Can you work these out from the model? Positions are in its coordinate system, mm. A direction names the side the tool comes from. Give positions to 0.01 mm unless a question says otherwise; leave off trailing zeros. Write each loop counter-clockwise with the first axis right and the second up, starting at its lowest first coordinate (ties: lowest second). Pieces come first, ordered by that corner, then holes.
from build123d import *

# Parameters (mm, degrees)
SKETCH1_R           = 76.2
SKETCH1_R_2         = 6.35
BOSS_EXTRUDE1_DEPTH = 2.413
SKETCH2_R           = 7.62
SKETCH2_R_2         = 6.35
BOSS_EXTRUDE3_DEPTH = 0.762
SKETCH4_R           = 76.257533764
CUT_EXTRUDE1_DEPTH  = 93.98
SKETCH5_R           = 1.016
CUT_EXTRUDE2_DEPTH  = 93.98


with BuildPart() as part:
    # Sketch1 → Boss-Extrude1 (new body)
    with BuildSketch(Plane.XY):
        Circle(SKETCH1_R)
        Circle(SKETCH1_R_2, mode=Mode.SUBTRACT)
    extrude(amount=BOSS_EXTRUDE1_DEPTH)

    # Sketch2 → Boss-Extrude3 (add)
    with BuildSketch(Plane.XY.offset(2.413)):
        with Locations(Location((0, 0, 0), (0, 0, 180))):
            Circle(SKETCH2_R)
        Circle(SKETCH2_R_2, mode=Mode.SUBTRACT)
    extrude(amount=BOSS_EXTRUDE3_DEPTH)

    # Sketch4 → Cut-Extrude1 (cut)
    with BuildSketch(Plane(origin=(0, 0, 0), x_dir=(-1, 0, 0), z_dir=(0, 0, -1))):
        Circle(SKETCH4_R)
        with BuildLine():
            Line((10.795, 13.97), (-10.795, 13.97))
            ThreePointArc((-10.795, 13.97), (-13.04006403, 14.89993597), (-13.97, 17.145))
            Line((-13.97, 17.145), (-13.97, 26.67))
            Line((-13.97, 26.67), (-18.20732863, 26.67))
            ThreePointArc((-18.20732863, 26.67), (-20.55370118, 20.591203739), (-23.658870968, 14.862752926))
            Line((-23.658870968, 14.862752926), (-4.737825132, -30.035944056))
            ThreePointArc((-4.737825132, -30.035944056), (0, -31.403636364), (4.737825132, -30.035944056))
            Line((4.737825132, -30.035944056), (23.658870968, 14.862752926))
            ThreePointArc((23.658870968, 14.862752926), (20.55370118, 20.591203739), (18.20732863, 26.67))
            Line((18.20732863, 26.67), (13.97, 26.67))
            Line((13.97, 26.67), (13.97, 17.145))
            ThreePointArc((13.97, 17.145), (13.04006403, 14.89993597), (10.795, 13.97))
        make_face(mode=Mode.SUBTRACT)
    extrude(amount=-CUT_EXTRUDE1_DEPTH, mode=Mode.SUBTRACT)

    # Sketch5 → Cut-Extrude2 (cut)
    with BuildSketch(Plane.XY.offset(2.413)):
        with Locations((-16.764, 23.241)):
            Circle(SKETCH5_R)
        with Locations((16.764, 23.241)):
            Circle(SKETCH5_R)
        with Locations((0, -28.575)):
            Circle(SKETCH5_R)
        with Locations((-5.5499, 8.7376)):
            Circle(SKETCH5_R)
        with Locations((5.5499, 8.7376)):
            Circle(SKETCH5_R)
    extrude(amount=-CUT_EXTRUDE2_DEPTH, mode=Mode.SUBTRACT)


solid = part.part
(1) Imagine slicing it at B-B, the plane y = 0. Write out the boundary of the cut face in (x, z) (3 decimals), plus the area to 3 significant figures.
Returned:
outline: (-17.395, 0) - (-6.35, 0) - (-6.35, 3.175) - (-7.62, 3.175) - (-7.62, 2.413) - (-17.395, 2.413) - close; (6.35, 0) - (17.395, 0) - (17.395, 2.413) - (7.62, 2.413) - (7.62, 3.175) - (6.35, 3.175) - close
area: 55.2 mm2
(2) Imagine slicing it at D-D, the plane x = -16.5. Write out the boundary of the cut face in (y, z), plus the area to 3 significant figures.
Returned:
outline: (-2.12, 0) - (22.26, 0) - (22.26, 2.41) - (-2.12, 2.41) - close; (24.22, 0) - (26.67, 0) - (26.67, 2.41) - (24.22, 2.41) - close
area: 64.7 mm2
(3) For faces 4 (the face through (-4.58, 9.04, 1.22)), 5 (the face through (0.992, -7.555, 2.789)), 6 (the face through (0, 13.97, 1)), which set-ups out of +Z, -Z, +X, -X, +Y, -Y let a thin tool reach every point of the face, with its end or its side?
Returned:
face 4: +Z, -Z
face 5: +Z
face 6: +Z, -Z, +Y
(4) Will these pins go through, and if not, where does the flat tip stop? P1, Ø1.9, axis at y = 21.5, z = 1, coming from the -X side; P2, Ø2, axis at x = -14.5, y = 18, coming from the -Z side; P3, Ø1, axis at y = -22, z = 2, coming from the -X side (3 decimals); P4, Ø5, axis at x = -17.5, y = 12, coming from the +Z side.
Returned:
P1: stops at x = -20.57
P2: stops at z = 0
P3: stops at x = -8.335
P4: stops at z = 2.41
(5) If we mould it in two halves opening along X, with no side actions, what happens to faces 1 (the face through (20.516, 20.674, 1.19)), 2 (the face through (17.7, 22.85, 1.22)), 3 (the face through (3, -6, 3.175))? For each: +X half, -X half, draft (parallel to the pull), parting line (faces both ways), or undercut.
Returned:
face 1: +X half
face 2: undercut
face 3: draft
(6) Imagine slicing it at C-C, the plane z = 1.3. Write out the boundary of the cut face in (x, y) (3 decimals), plus the area to 3 significant figures.
Returned:
outline: (-23.659, 14.863) - (-4.738, -30.036) arc R8.89 ccw to (4.738, -30.036) - (23.659, 14.863) arc R50.8 cw to (18.207, 26.67) - (13.97, 26.67) - (13.97, 17.145) arc R3.175 cw to (10.795, 13.97) - (-10.795, 13.97) arc R3.175 cw to (-13.97, 17.145) - (-13.97, 26.67) - (-18.207, 26.67) arc R50.8 cw to start; hole circle Ø2.032 at (-16.764, 23.241); hole circle Ø2.032 at (-5.55, 8.738); hole circle Ø12.7 at (0, 0); hole circle Ø2.032 at (0, -28.575); hole circle Ø2.032 at (5.55, 8.738); hole circle Ø2.032 at (16.764, 23.241)
area: 1,280 mm2
(7) If I drill on L1, parallel to X at y = 23.5, z = 0.55; L2, parallel to Z at x = 16, y = 5.5; L3, parallel to X at y = -5.5, z = 1.55, over which ranges is the centre line in solid material (lowest first)?
Returned:
L1: x = -19.32 to -17.75, -15.78 to -13.97, 13.97 to 15.78, 17.75 to 19.32
L2: z = 0 to 2.41
L3: x = -15.08 to -3.17, 3.17 to 15.08
(8) Imagine slicing it at A-A, the plane x = 0. Write out the boundary of the cut face in (y, z) (3 decimals).
Returned:
outline: (-31.404, 0) - (-29.591, 0) - (-29.591, 2.413) - (-31.404, 2.413) - close; (-27.559, 0) - (-6.35, 0) - (-6.35, 3.175) - (-7.62, 3.175) - (-7.62, 2.413) - (-27.559, 2.413) - close; (6.35, 0) - (13.97, 0) - (13.97, 2.413) - (7.62, 2.413) - (7.62, 3.175) - (6.35, 3.175) - close
